```python
from build123d import *

# Parameters (mm, degrees)
SKETCH1_W               = 34
SKETCH1_H               = 18
BOSS_EXTRUDE1_DEPTH     = 2.032
SKETCH2_R               = 0.762
BOSS_EXTRUDE2_DEPTH     = 1.524
SKETCH4_W               = 2.032
SKETCH4_H               = 22.225
BOSS_EXTRUDE3_DEPTH     = 11.43
SKETCH3_R               = 3.175
SKETCH3_R_2             = 2.0574
CUT_EXTRUDE1_DEPTH      = 1
CUT_EXTRUDE1_DEPTH_BACK = 35
SKETCH5_W               = 12.0904
SKETCH5_H               = 9.9568
CUT_EXTRUDE2_DEPTH      = 2.032


with BuildPart() as part:
    # Sketch1 → Boss-Extrude1 (new body)
    with BuildSketch(Plane(origin=(0, 0, 0), x_dir=(1, 0, 0), z_dir=(0, 1, 0))):
        Rectangle(SKETCH1_W, SKETCH1_H)
    extrude(amount=BOSS_EXTRUDE1_DEPTH)

    # Sketch2 → Boss-Extrude2 (add)
    with BuildSketch(Plane(origin=(0, 0, 0), x_dir=(-1, 0, 0), z_dir=(0, -1, 0))):
        with Locations((-15.476, 5.224)):
            Circle(SKETCH2_R)
        with Locations((-15.476, -7.222)):
            Circle(SKETCH2_R)
        with Locations((15.476, -7.222)):
            Circle(SKETCH2_R)
        with Locations((15.476, 6.494)):
            Circle(SKETCH2_R)
    extrude(amount=BOSS_EXTRUDE2_DEPTH)

    # Sketch4 → Boss-Extrude3 (add)
    with BuildSketch(Plane(origin=(0, 2.032, 0), x_dir=(1, 0, 0), z_dir=(0, 1, 0))):
        with Locations((-12.174, -2.1125)):
            Rectangle(SKETCH4_W, SKETCH4_H)
        with Locations((12.174, -2.1125)):
            Rectangle(SKETCH4_W, SKETCH4_H)
    extrude(amount=BOSS_EXTRUDE3_DEPTH)

    # Sketch3 → Cut-Extrude1 (cut, two sides)
    with BuildSketch(Plane.ZY.offset(17)) as cut_extrude1_sk:
        with Locations((-2.0658, 5.7912)):
            Circle(SKETCH3_R)
        with Locations((8.276585961, 7.0104)):
            Circle(SKETCH3_R_2)
    extrude(amount=CUT_EXTRUDE1_DEPTH, mode=Mode.SUBTRACT)
    extrude(cut_extrude1_sk.sketch, amount=-CUT_EXTRUDE1_DEPTH_BACK, mode=Mode.SUBTRACT)

    # Sketch5 → Cut-Extrude2 (cut)
    with BuildSketch(Plane(origin=(13.19, 0, 0), x_dir=(0, 0, -1), z_dir=(1, 0, 0))):
        with Locations((-8.276585961, 7.0104)):
            Rectangle(SKETCH5_W, SKETCH5_H)
    extrude(amount=-CUT_EXTRUDE2_DEPTH, mode=Mode.SUBTRACT)


solid = part.part
```
CAD build for the part. Positions are in the model's coordinates, mm. A direction names the side the tool comes from. Coordinates: 2 decimals unless noted, no trailing zeros. Order: outer loops, then holes, each group sorted by start corner. A loop starts at its lowest first (then second) coordinate and runs counter-clockwise, first axis right, second up.
(1) Drill centre lines: L1, parallel to X at y = 8, z = -5.25; L2, parallel to Y at x = 0.5, z = 2.5; L3, parallel to X at y = 2.5, z = 10. Where is each one in solid material? Low to high.
Solution:
L1: x = -13.19 to -11.16, 11.16 to 13.19
L2: y = 0 to 2.03
L3: x = -13.19 to -11.16
(2) Saw through at B-B, the plane x = 12. Write the cut outline in (y, z) (3 decimals).
Solution:
outline: (0, -9) - (13.462, -9) - (13.462, 13.225) - (11.989, 13.225) - (11.989, 2.231) - (2.032, 2.231) - (2.032, 9) - (0, 9) - close; hole circle Ø6.35 at (5.791, -2.066)
(3) Saw through at C-C, the plane y = 7.5. Write the cut outline in (x, z) (3 decimals), and give its area (3 significant figures).
Solution:
outline: (-13.19, -9) - (-11.158, -9) - (-11.158, -4.742) - (-13.19, -4.742) - close; (-13.19, 0.61) - (-11.158, 0.61) - (-11.158, 6.278) - (-13.19, 6.278) - close; (-13.19, 10.275) - (-11.158, 10.275) - (-11.158, 13.225) - (-13.19, 13.225) - close; (11.158, -9) - (13.19, -9) - (13.19, -4.742) - (11.158, -4.742) - close; (11.158, 0.61) - (13.19, 0.61) - (13.19, 2.231) - (11.158, 2.231) - close
area: 38.1 mm2
(4) Saw through at A-A, the plane y = 4.25. Write the cut outline in (x, z) (3 decimals), and give its area (3 significant figures).
Solution:
outline: (-13.19, -9) - (-11.158, -9) - (-11.158, -4.842) - (-13.19, -4.842) - close; (-13.19, 0.71) - (-11.158, 0.71) - (-11.158, 13.225) - (-13.19, 13.225) - close; (11.158, -9) - (13.19, -9) - (13.19, -4.842) - (11.158, -4.842) - close; (11.158, 0.71) - (13.19, 0.71) - (13.19, 2.231) - (11.158, 2.231) - close
area: 45.4 mm2
(5) Mould opens along Z. For faces 1 (the face through (3, 2.032, 0)), 2 (the face through (12, 13, 13.225)), 3 (the face through (-15.828, -0.751, 7.898)) say: released by +Z, released by -Z, zero draft, split by the parting line, or undercut.
Solution:
face 1: zero draft
face 2: released by +Z
face 3: undercut
(6) Which spindle directions (+Z, -Z, +X, -X, +Y, -Y) get a long thin tool onto all of the face, cutting with end or side? Do faces 4 (the face through (11.158, 9, -3)), 5 (the face through (12, 7, 2.231)), 6 (the face through (-13.19, 8, 2)). Say none if no direction does.
Solution:
face 4: +Z, -Z, +Y
face 5: +Z, +X
face 6: +Z, -Z, -X, +Y
(7) Saw through at D-D, the plane y = 1.5. Write the cut outline in (x, z).
Solution:
outline: (-17, -9) - (17, -9) - (17, 9) - (-17, 9) - close
(8) Pin check, flat tips, straight feed: pin 1 Ø5.5 at (y, z) = (7.5, 6.5) entering from +X; pin 2 Ø2 at (x, z) = (12, 6) entering from -Y; pin 3 Ø10 at (x, z) = (-3, -1) entering from +Y; pin 4 Ø5 at (y, z) = (5.79, -2.07) entering from +X. Stop position of each tip, or through.
Solution:
pin 1: stops at x = -11.16
pin 2: stops at y = 0
pin 3: stops at y = 2.03
pin 4: passes through
